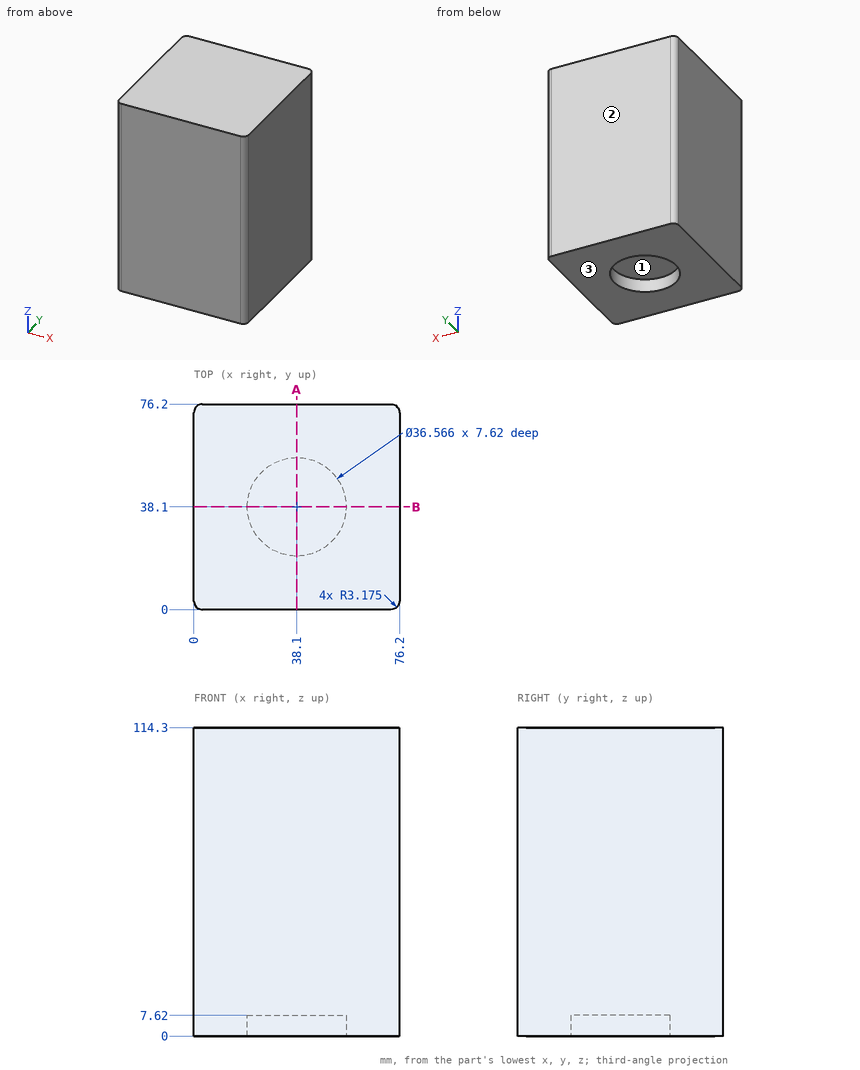
Here's the drawing with two shaded views (mm, measured from the low corner). I have some questions. Give positions to 0.01 mm unless a question says otherwise; leave off trailing zeros. Write each loop counter-clockwise with the first axis right and the second up, starting at its lowest first coordinate (ties: lowest second). Pieces come first, ordered by that corner, then holes. Notation, with made-up numbers: (71.5, 73.5) -> (103.5, 73.5) arc R25 ccw to (103.5, 85.5) -> close; hole circle Ø8 at (1, -33). An arc over 180 degrees is marked (long way). Use one line per item in the form item = value. Start each with the question number.
1. Imagine slicing it at A-A on x = 38.1. List the corners of the cut face in (y, z) for me, plus the area to 3 significant figures.
2. Thinking about a two-plate mould opening in Y: for the marked faces 1, 2 and 3, which applies, +Y half, -Y half, draft (parallel to the pull), parting line (faces both ways), or undercut?
3. Will this pin go through, and if not, where does the flat tip stop? pin 1 Ø18.5 at (x, y) = (42.5, 41) entering from -Z.
4. If I drill on L1, parallel to X at y = 38, z = 5; L2, parallel to Z at x = 39, y = 38.5, over which ranges is the centre line in solid material (lowest first)?
Entries:
q1.outline = (0, 0) -> (19.82, 0) -> (19.82, 7.62) -> (56.38, 7.62) -> (56.38, 0) -> (76.2, 0) -> (76.2, 114.3) -> (0, 114.3) -> close
q1.area = 8,430 mm²
q2.face_1 = undercut
q2.face_2 = +Y half
q2.face_3 = draft
q3.pin_1 = 7.62
q4.L1 = 0 to 19.82, 56.38 to 76.2
q4.L2 = 7.62 to 114.3
